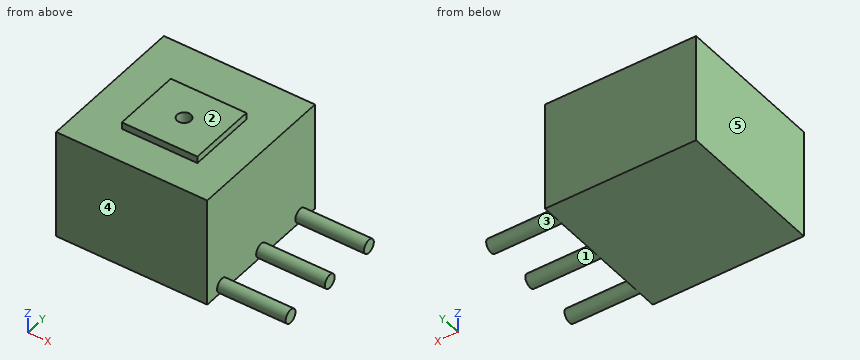
from build123d import *

# Parameters (mm, degrees)
SKETCH_W     = 11
SKETCH_H     = 11
PAD_DEPTH    = 8
SKETCH001_R  = 0.5
PAD001_DEPTH = 5
SKETCH002_W  = 5.5
SKETCH002_H  = 5
PAD002_DEPTH = 0.5
SKETCH003_R  = 0.5
POCKET_DEPTH = 2


with BuildPart() as part:
    # Sketch → Pad (new body)
    with BuildSketch(Plane.XY):
        Rectangle(SKETCH_W, SKETCH_H)
    extrude(amount=PAD_DEPTH)

    # Sketch001 (on Face2 of Pad) → Pad001 (join)
    with BuildSketch(Plane.YZ.offset(5.5)):
        with Locations((-4, 0.5)):
            Circle(SKETCH001_R)
        with Locations((0, 0.5)):
            Circle(SKETCH001_R)
        with Locations((4, 0.5)):
            Circle(SKETCH001_R)
    extrude(amount=PAD001_DEPTH)

    # Sketch002 (on Face5 of Pad001) → Pad002 (join)
    with BuildSketch(Plane.XY.offset(8)):
        with Locations((0.25, -0.5)):
            Rectangle(SKETCH002_W, SKETCH002_H)
    extrude(amount=PAD002_DEPTH)

    # Sketch003 (on Face17 of Pad002) → Pocket (cut)
    with BuildSketch(Plane.XY.offset(8.5)):
        with Locations((0.25, -0.5)):
            Circle(SKETCH003_R)
    extrude(amount=-POCKET_DEPTH, mode=Mode.SUBTRACT)


solid = part.part
Check sheet for the modelled part. Datum: model origin and axes. Units: mm. Face numbers are marked on the shaded views. A direction names the side the tool comes from. Give positions to 0.01 mm unless a question says otherwise; leave off trailing zeros. Loops run counter-clockwise (first coordinate to the right, second up) from the corner with the lowest first, then second, coordinate; pieces in that order, holes last. Notation, with made-up numbers: M 13.5,80.5 L 71.5,80.5 A6 ccw 71.5,84.5 Z; hole C -38,72 d1. An arc over 180 degrees is marked long. Answer as a JSON object with one key per item and string values. Group by question number.
Q1. Cross-section at D-D on z = 0.5. Record the cut outline in (x, y), then the cut area to 3 significant figures.
Q2. Go/stop test with flat-tipped pins: P1, Ø0.6, axis at y = -0.5, z = 8.5, coming from the +X side; P2, Ø0.6, axis at y = -1, z = 8.5, coming from the -X side; P3, Ø2, axis at x = -3.5, y = -2.5, coming from the -Z side. Record where each tip stops, or that it passes through.
Q3. Access from +Z, -Z, +X, -X, +Y, -Y to the whole of each face (thin tool, end or side, straight path). Record for the marked faces 1 and 2.
Q4. Cross-section at A-A on x = 2.5. Record the cut outline in (y, z), then the cut area to 3 significant figures.
Q5. Release check for a two-part mould opening along Y. For the marked faces 3, 4 and 5 record: released by +Y, released by -Y, zero draft, split by the parting line, or undercut.
Q6. Cross-section at B-B on y = 1.25. Record the cut outline in (x, z).
Q7. Material ranges on line 1 along Y through (x, z) = (0.25, 7.55); line 2 along Z through (x, y) = (-3.5, -3.75); line 3 along X through (y, z) = (3.5, 6.75), recorded low to high. Write a range as [from, to].
Q8. Cross-section at C-C on x = 6.75. Record the cut outline in (y, z).
Evaluation:
{
 "1": {"outline": "M -5.5,-5.5 L 5.5,-5.5 L 5.5,-4.5 L 10.5,-4.5 L 10.5,-3.5 L 5.5,-3.5 L 5.5,-0.5 L 10.5,-0.5 L 10.5,0.5 L 5.5,0.5 L 5.5,3.5 L 10.5,3.5 L 10.5,4.5 L 5.5,4.5 L 5.5,5.5 L -5.5,5.5 Z", "area": "136 mm2"},
 "2": {"P1": "stops at x = 3", "P2": "stops at x = -2.5", "P3": "stops at z = 0"},
 "3": {"face 1": "+X", "face 2": "+Z, +X, -X, +Y, -Y"},
 "4": {"outline": "M -5.5,0 L 5.5,0 L 5.5,8 L 2,8 L 2,8.5 L -3,8.5 L -3,8 L -5.5,8 Z", "area": "90.5 mm2"},
 "5": {"face 3": "undercut", "face 4": "released by -Y", "face 5": "zero draft"},
 "6": {"outline": "M -5.5,0 L 5.5,0 L 5.5,8 L 3,8 L 3,8.5 L -2.5,8.5 L -2.5,8 L -5.5,8 Z"},
 "7": {"line 1": "y = [-5.5, -1], [0, 5.5]", "line 2": "z = [0, 8]", "line 3": "x = [-5.5, 5.5]"},
 "8": {"outline": "C -4,0.5 d1; C 0,0.5 d1; C 4,0.5 d1"}
}
